Answer from the drawing. Dimensions are ordinates in mm from the lowest x, y and z of the part. A direction names the side the tool comes from. Coordinates: 2 decimals unless noted, no trailing zeros. Order: outer loops, then holes, each group sorted by start corner. A loop starts at its lowest first (then second) coordinate and runs counter-clockwise, first axis right, second up. Notation, with made-up numbers: (77, 34.25) - (131, 34.25) arc R13 cw to (131, 52.25) - close; hole circle Ø7 at (48, 10.25). An arc over 180 degrees is marked (long way). Use a Markdown table: item, result. Add a question column.
Item 1: A flat-ended cylindrical pin translates along its axis: P1, Ø4, axis at x = 8.5, y = 7, coming from the -Z side. Find the tip coordinate at first contact, or state that the pin passes through.
Item 2: Find the intervals of material crossed by line 1 along Y through (x, z) = (3.25, 0.75); line 2 along X through (y, z) = (11.25, 7); line 3 along X through (y, z) = (8, 3.25), in increasing order.
Item 3: For the marked faces 1 and 2, determine the directions among +Z, -Z, +X, -X, +Y, -Y from which every point of the face is accessible in a straight line to the end or side of a thin tool.
Item 4: The mould has two halves that part along Y. Classify the marked faces 3, 4 and 5: released by +Y, released by -Y, zero draft, split by the parting line, or undercut.
Item 5: The part is cut by section B-B, the plane z = 6.25. Give the vertices of the cut face in (x, y), then the cut area to 4 significant figures.
Item 6: The part is cut by section C-C, the plane z = 11. Give the vertices of the cut face in (x, y).
Item 7: The part is cut by section A-A, the plane x = 10.25. Give the vertices of the cut face in (y, z).
Item 8: The part is cut by section D-D, the plane x = 6.25. Give the vertices of the cut face in (y, z), then the cut area to 4 significant figures.
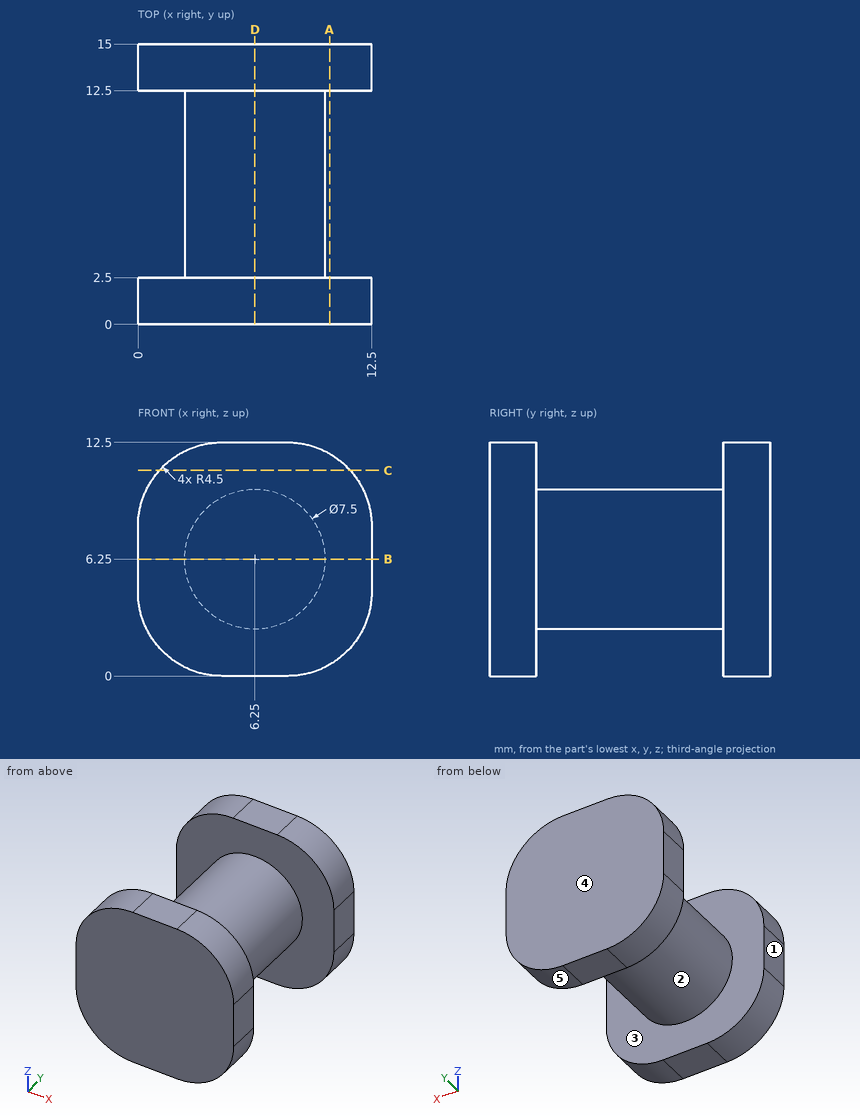
Solution:
| question | item | result |
|---|---|---|
| 1 | P1 | stops at z = 2.51 |
| 2 | line 1 | y = 0 to 2.5, 12.5 to 15 |
| 2 | line 2 | x = 2.58 to 9.92 |
| 2 | line 3 | x = 4 to 8.5 |
| 3 | face 1 | +Z, -Z, -X, +Y, -Y |
| 3 | face 2 | none |
| 4 | face 3 | undercut |
| 4 | face 4 | released by +Y |
| 4 | face 5 | zero draft |
| 5 | outline | (0, 0) - (12.5, 0) - (12.5, 2.5) - (10, 2.5) - (10, 12.5) - (12.5, 12.5) - (12.5, 15) - (0, 15) - (0, 12.5) - (2.5, 12.5) - (2.5, 2.5) - (0, 2.5) - close |
| 5 | area | 137.5 mm2 |
| 6 | outline | (1.15, 0) - (11.35, 0) - (11.35, 2.5) - (1.15, 2.5) - close; (1.15, 12.5) - (11.35, 12.5) - (11.35, 15) - (1.15, 15) - close |
| 7 | outline | (0, 0.6) - (2.5, 0.6) - (2.5, 11.9) - (0, 11.9) - close; (12.5, 0.6) - (15, 0.6) - (15, 11.9) - (12.5, 11.9) - close |
| 8 | outline | (0, 0) - (2.5, 0) - (2.5, 2.5) - (12.5, 2.5) - (12.5, 0) - (15, 0) - (15, 12.5) - (12.5, 12.5) - (12.5, 10) - (2.5, 10) - (2.5, 12.5) - (0, 12.5) - close |
| 8 | area | 137.5 mm2 |
